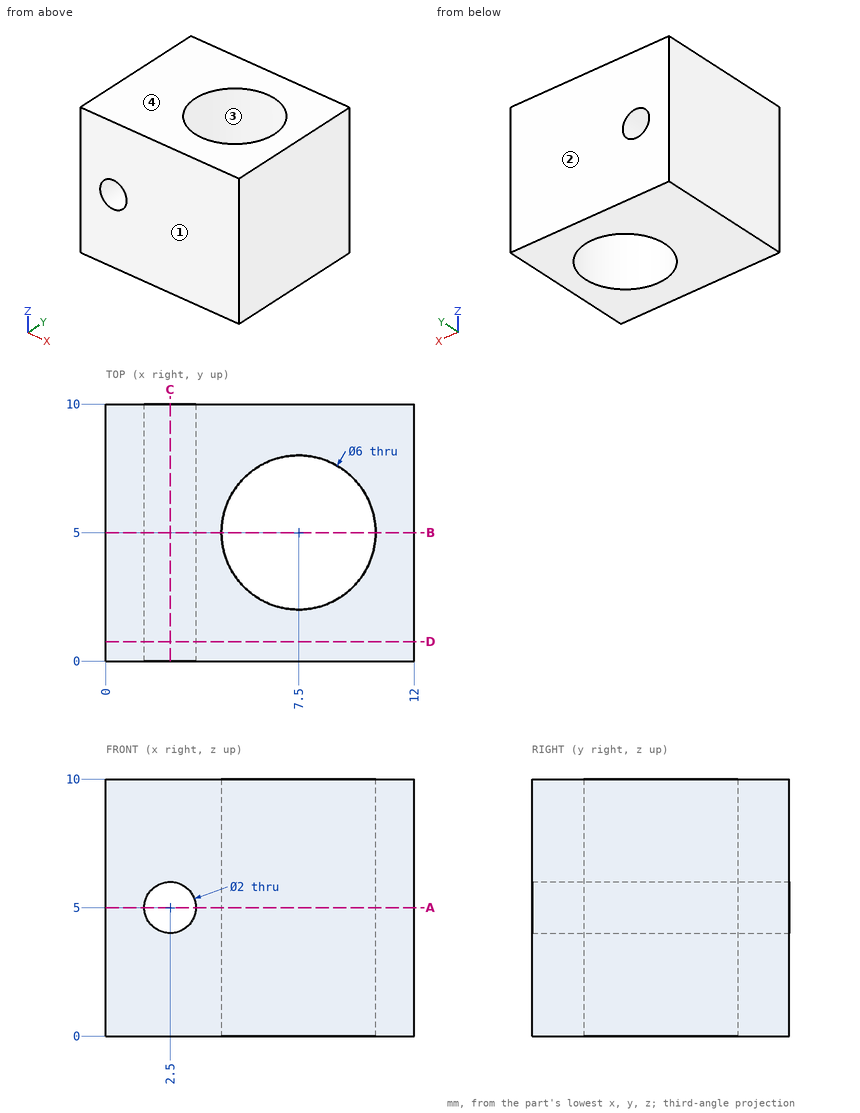
Part print with two shaded views. Sizes in mm from the minimum x, y, z corner. Coordinates: 2 decimals unless noted, no trailing zeros. Order: outer loops, then holes, each group sorted by start corner. A loop starts at its lowest first (then second) coordinate and runs counter-clockwise, first axis right, second up. Notation, with made-up numbers: M 44.5,-20 L 81.5,-20 A19 cw 81.5,13 Z; hole C -14.75,41 d1. An arc over 180 degrees is marked long. One line per question, with ' | ' between items. Start each with the question number.
1. Cut at A-A (z = 5). Write the cut outline in (x, y).
2. Mould opens along Y. For the marked faces 1, 2, 3 and 4 say: +Y half, -Y half, draft (parallel to the pull), parting line (faces both ways), or undercut.
3. Cut at C-C (x = 2.5). Write the cut outline in (y, z).
4. Flat gauge pin, fed straight in: P1, Ø1, axis at y = 1.5, z = 7, coming from the -X side. Where does the tip first touch, or does it go through?
5. Wall check: line 1 along X through (y, z) = (5, 2.5); line 2 along Z through (x, y) = (2.5, 4.5); line 3 along X through (y, z) = (5.75, 5). Give the ranges that are in metal, low to high. Write a range as [from, to].
6. Cut at D-D (y = 0.75). Write the cut outline in (x, z), plus the area to 3 significant figures.
7. Cut at B-B (y = 5). Write the cut outline in (x, z), plus the area to 3 significant figures.
The answers:
1) outline: M 0,0 L 1.5,0 L 1.5,10 L 0,10 Z; M 3.5,0 L 12,0 L 12,10 L 3.5,10 Z; hole C 7.5,5 d6
2) face 1: -Y half | face 2: +Y half | face 3: undercut | face 4: draft
3) outline: M 0,0 L 10,0 L 10,4 L 0,4 Z; M 0,6 L 10,6 L 10,10 L 0,10 Z
4) P1: stops at x = 0
5) line 1: x = [0, 4.5], [10.5, 12] | line 2: z = [0, 4], [6, 10] | line 3: x = [0, 1.5], [3.5, 4.6], [10.4, 12]
6) outline: M 0,0 L 12,0 L 12,10 L 0,10 Z; hole C 2.5,5 d2 | area: 117 mm2
7) outline: M 0,0 L 4.5,0 L 4.5,10 L 0,10 Z; M 10.5,0 L 12,0 L 12,10 L 10.5,10 Z; hole C 2.5,5 d2 | area: 56.9 mm2
